```python
from build123d import *

# Parameters (mm, degrees)
SKETCH2_R          = 2.5
CUT_EXTRUDE1_DEPTH = 79.914255008


with BuildPart() as part:
    # Sketch1 → Revolve2 (revolve)
    with BuildSketch(Plane.XY, mode=Mode.PRIVATE) as revolve2_sk:
        with BuildLine():
            Line((-13.637604781, 9), (21.379821609, 9))
            Line((21.379821609, 9), (21.379821609, 15))
            Line((21.379821609, 15), (5.627244289, 15))
            ThreePointArc((5.627244289, 15), (3.505923946, 15.878679656), (2.627244289, 18))
            Line((2.627244289, 18), (2.627244289, 32))
            ThreePointArc((2.627244289, 32), (3.505923946, 34.121320344), (5.627244289, 35))
            Line((5.627244289, 35), (6.362395219, 35))
            Line((6.362395219, 35), (6.362395219, 45.687700042))
            Line((6.362395219, 45.687700042), (2.494845361, 45.687700042))
            Line((2.494845361, 45.687700042), (2.494845361, 43))
            ThreePointArc((2.494845361, 43), (1.616165704, 40.878679656), (-0.505154639, 40))
            Line((-0.505154639, 40), (-4.505154639, 40))
            ThreePointArc((-4.505154639, 40), (-6.626474983, 40.878679656), (-7.505154639, 43))
            Line((-7.505154639, 43), (-7.505154639, 45))
            Line((-7.505154639, 45), (-13.637604781, 45))
            Line((-13.637604781, 45), (-13.637604781, 9))
        make_face()
    revolve(revolve2_sk.sketch.rotate(Axis((-27.298969072, 0, 0), (1, 0, 0)), 90), axis=Axis((-27.298969072, 0, 0), (1, 0, 0)))

    # Sketch2 → Cut-Extrude1 (cut, through all)
    with BuildSketch(Plane(origin=(0, 15, 0), x_dir=(1, 0, 0), z_dir=(0, 1, 0))):
        with Locations(Location((11.379821609, 0, 0), (0, 0, 270))):
            Circle(SKETCH2_R)
    extrude(amount=-CUT_EXTRUDE1_DEPTH, mode=Mode.SUBTRACT)


solid = part.part
```
Check sheet for the modelled part. Datum: model origin and axes. Units: mm. A direction names the side the tool comes from. Round coordinates to 2 decimals unless told otherwise and drop trailing zeros. Answer in a Markdown table with one row per item.
(1) Set-up check for faces 5 (the cylindrical face through (13.393, 14.643, -3.252)), 6 (the cylindrical face through (-2.53, -1.76, -39.96)), 7 (the cylindrical face through (12.131, -11.777, 2.385)), 8 (the cylindrical face through (-10.614, 39.923, 20.765)): record each of +Z, -Z, +X, -X, +Y, -Y from which the full face is reachable in a straight line by a thin tool's end or side.
Findings:
| item | result |
|---|---|
| face 5 | +X |
| face 6 | none |
| face 7 | +Y, -Y |
| face 8 | -X |
(2) Gauge pin test, flat ends, axial feed: pin 1 (4 mm diameter, centred on x = 9, y = -5.5, fed in from -Z); pin 2 (6 mm diameter, centred on x = 11.38, z = 0, fed in from +Y); pin 3 (10 mm diameter, centred on x = 1.5, y = -10, fed in from -Z). Record the tip position at first contact, or that the pin passes through.
Findings:
| item | result |
|---|---|
| pin 1 | stops at z = -14.59 |
| pin 2 | stops at y = 15 |
| pin 3 | stops at z = -45.4 |
(3) Draft check along Y on faces 1 (the flat face through (21.38, 6.5, -6.5)), 2 (the cylindrical face through (4.402, 40.533, 21.082)), 3 (the cylindrical face through (4.116, -2.703, 8.584)), 4 (the flat face through (2.627, 14, -14)). Enter one of: +Y half, -Y half, draft (parallel to the pull), parting line (faces both ways), or undercut.
Findings:
| item | result |
|---|---|
| face 1 | draft |
| face 2 | parting line |
| face 3 | undercut |
| face 4 | undercut |
(4) Section check B-B on z = 0. Give the number of separate pieces and of enclosed holes in the cut face, plus the area to 3 significant figures.
Findings:
| item | result |
|---|---|
| separate pieces | 4 |
| enclosed holes | 0 |
| area | 1,330 mm^2 |
(5) Material ranges on line 1 along Y through (x, z) = (6.15, 0); line 2 along Y through (x, z) = (-3, 0); line 3 along X through (y, z) = (-38, 3.5), recorded low to high. Write a range as from..to.
Findings:
| item | result |
|---|---|
| line 1 | y = -45.69..-35, -15..-9, 9..15, 35..45.69 |
| line 2 | y = -40..-9, 9..40 |
| line 3 | x = -13.64..6.36 |
